Work out the finished part from the listing and answer in its coordinate system (mm). A direction names the side the tool comes from. Round coordinates to 2 decimals unless told otherwise and drop trailing zeros. Write each loop counter-clockwise with the first axis right and the second up, starting at its lowest first coordinate (ties: lowest second). Pieces come first, ordered by that corner, then holes. Notation, with made-up numbers: M 20.5,-25.5 L 41.5,-25.5 A26 ccw 41.5,5.5 Z; hole C -1.75,5 d5. An arc over 180 degrees is marked long. Answer in a Markdown table with one row per item.
```python
from build123d import *

# Parameters (mm, degrees)
EXTRUDE_1_DEPTH     = 12
SKETCH_2_R          = 1.6
CUT_EXTRUDE_1_DEPTH = 45.2
CHAMFER_1_SIZE      = 2
SKETCH_4_R          = 1.5
CUT_EXTRUDE_2_DEPTH = 52.15662225
SKETCH_6_W          = 26.1795091
SKETCH_6_H          = 41
CUT_EXTRUDE_3_DEPTH = 10
CHAMFER_2_SIZE      = 4
CHAMFER_4_SIZE      = 5


with BuildPart() as part:
    # Эскиз1 → Бобышка-Вытянуть1 (new, symmetric)
    with BuildSketch(Plane.XY):
        Polygon((0, 0), (0, 48), (1.5, 48), (1.5, 1.5), (13, 1.5), (13, 0), align=None)
    extrude(amount=EXTRUDE_1_DEPTH, both=True)

    # Эскиз2 → Вырез-Вытянуть1 (cut)
    with BuildSketch(Plane(origin=(0, 1.5, 0), x_dir=(1, 0, 0), z_dir=(0, 1, 0))):
        with Locations(Location((9, 0, 0), (0, 0, 270))):
            Circle(SKETCH_2_R)
        with Locations(Location((9, -8, 0), (0, 0, 270))):
            Circle(SKETCH_2_R)
        with Locations(Location((9, 8, 0), (0, 0, 270))):
            Circle(SKETCH_2_R)
    extrude(amount=-CUT_EXTRUDE_1_DEPTH, mode=Mode.SUBTRACT)

    # Фаска1
    chamfer_1_edges = [part.edges().sort_by_distance(p)[0] for p in [
        (13, 0.75, 12),
        (13, 0.75, -12),
    ]]
    chamfer(chamfer_1_edges, length=CHAMFER_1_SIZE)

    # Эскиз4 → Вырез-Вытянуть2 (cut, through all)
    with BuildSketch(Plane.ZY):
        with Locations((0, 42.5)):
            Circle(SKETCH_4_R)
        with Locations((0, 5.5)):
            Circle(SKETCH_4_R)
    extrude(amount=-CUT_EXTRUDE_2_DEPTH, mode=Mode.SUBTRACT)

    # Эскиз6 → Вырез-Вытянуть3 (cut)
    with BuildSketch(Plane.ZY):
        Polygon((7, 72.5), (7, 42.5), (33.1795091, 42.5), (33.38840833, 42.5), (33.38840833, 72.5), align=None)
        with Locations((20.08975455, 22)):
            Rectangle(SKETCH_6_W, SKETCH_6_H)
        with Locations((-20.08975455, 22)):
            Rectangle(SKETCH_6_W, SKETCH_6_H)
        Polygon((-33.38840833, 42.5), (-33.1795091, 42.5), (-7, 42.5), (-7, 72.5), (-33.38840833, 72.5), align=None)
    extrude(amount=-CUT_EXTRUDE_3_DEPTH, mode=Mode.SUBTRACT)

    # Фаска2
    chamfer_2_edges = [part.edges().sort_by_distance(p)[0] for p in [
        (0.75, 48, -7),
        (0.75, 48, 7),
    ]]
    chamfer(chamfer_2_edges, length=CHAMFER_2_SIZE)

    # Фаска4
    chamfer_4_edges = [part.edges().sort_by_distance(p)[0] for p in [
        (0.75, 1.5, 7),
        (0.75, 1.5, -7),
    ]]
    chamfer(chamfer_4_edges, length=CHAMFER_4_SIZE - 0.0001)  # a hair under: the kernel refuses the full size


solid = part.part
```
1. The part is cut by section A-A (z = 0). Determine the outline of the cut face in (x, y), plus the area to 4 significant figures.
Calculated:
| item | result |
|---|---|
| outline | M 0,0 L 7.4,0 L 7.4,1.5 L 1.5,1.5 L 1.5,4 L 0,4 Z; M 0,7 L 1.5,7 L 1.5,41 L 0,41 Z; M 0,44 L 1.5,44 L 1.5,48 L 0,48 Z; M 10.6,0 L 13,0 L 13,1.5 L 10.6,1.5 Z |
| area | 75.45 mm² |
2. Determine the mould class of faces 1 (the flat face through (1, 26, 7)), 2 (the cylindrical face through (7.44, 0.76, -8.35)), 3 (the flat face through (13, 1, 0)) for opening direction X: released by +X, released by -X, zero draft, split by the parting line, or undercut.
Calculated:
| item | result |
|---|---|
| face 1 | zero draft |
| face 2 | undercut |
| face 3 | released by +X |
3. The part is cut by section D-D (z = -8). Determine the outline of the cut face in (x, y), plus the area to 3 significant figures.
Calculated:
| item | result |
|---|---|
| outline | M 0,0 L 7.4,0 L 7.4,1.5 L 1.5,1.5 L 1.5,5.5 L 0,5.5 Z; M 10.6,0 L 13,0 L 13,1.5 L 10.6,1.5 Z |
| area | 20.7 mm² |
4. Consider line 1 along Y through (x, z) = (0.55, 0); line 2 along X through (y, z) = (1.15, -8); line 3 along Y through (x, z) = (11.25, 5.5). Determine where each line is inside the solid, lowest interval first. Write a range as from..to.
Calculated:
| item | result |
|---|---|
| line 1 | y = 0..4, 7..41, 44..48 |
| line 2 | x = 0..7.4, 10.6..13 |
| line 3 | y = 0..1.5 |
5. A tool of negligible diameter and unlimited length cuts with its end or side. For faces 4 (the flat face through (1, 25, -7)), 5 (the flat face through (12, 1, -11)), 6 (the flat face through (1.5, 25, 0)), from which of +Z, -Z, +X, -X, +Y, -Y can it reach the whole face along a straight path? Write none if from no direction.
Calculated:
| item | result |
|---|---|
| face 4 | -Z, +X, -X, +Y |
| face 5 | -Z, +X, +Y, -Y |
| face 6 | +Z, -Z, +X, +Y |
6. The part is cut by section C-C (y = 5.5). Determine the outline of the cut face in (x, z), plus the area to 3 significant figures.
Calculated:
| item | result |
|---|---|
| outline | M 0,-8 L 1.5,-8 L 1.5,-1.5 L 0,-1.5 Z; M 0,1.5 L 1.5,1.5 L 1.5,8 L 0,8 Z |
| area | 19.5 mm² |
7. The part is cut by section B-B (x = 9). Determine the outline of the cut face in (y, z), plus the area to 3 significant figures.
Calculated:
| item | result |
|---|---|
| outline | M 0,-12 L 1.5,-12 L 1.5,-9.6 L 0,-9.6 Z; M 0,-6.4 L 1.5,-6.4 L 1.5,-1.6 L 0,-1.6 Z; M 0,1.6 L 1.5,1.6 L 1.5,6.4 L 0,6.4 Z; M 0,9.6 L 1.5,9.6 L 1.5,12 L 0,12 Z |
| area | 21.6 mm² |
8. Given pin 1 (4 mm diameter, centred on x = 9, z = 8, fed in from +Y); pin 2 (0.8 mm diameter, centred on x = 1, y = 24, fed in from -Z); pin 3 (3.5 mm diameter, centred on y = 5.5, z = 0, fed in from +X), each flat-ended and moving along its own axis, determine where each tip first touches the part or whether it passes through.
Calculated:
| item | result |
|---|---|
| pin 1 | stops at y = 1.5 |
| pin 2 | stops at z = -7 |
| pin 3 | stops at x = 1.5 |
